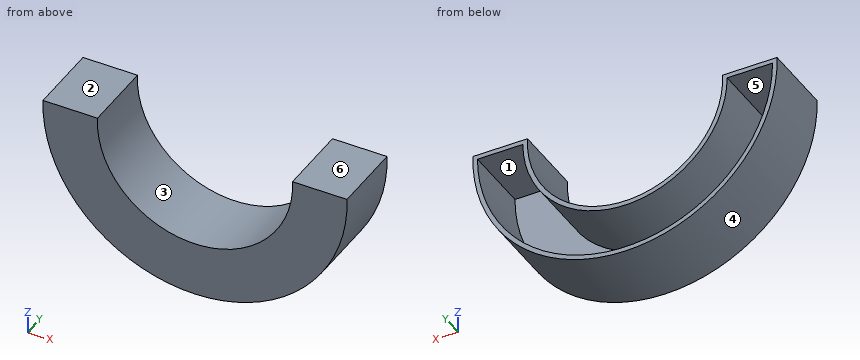
from build123d import *

# Parameters (mm, degrees)
BOSS_EXTRUDE1_DEPTH = 6
BOSS_EXTRUDE2_DEPTH = 0.4


with BuildPart() as part:
    # Sketch3 → Boss-Extrude1 (new body)
    with BuildSketch(Plane(origin=(0, 0, 0), x_dir=(1, 0, 0), z_dir=(0, 1, 0))):
        with BuildLine():
            Line((8.590692638, -0.4), (13.39402852, -0.4))
            ThreePointArc((13.39402852, -0.4), (0, 13.4), (-13.39402852, -0.4))
            Line((-13.39402852, -0.4), (-8.590692638, -0.4))
            ThreePointArc((-8.590692638, -0.4), (0, 8.6), (8.590692638, -0.4))
        make_face()
        with BuildLine():
            Line((9, 0), (13, 0))
            ThreePointArc((13, 0), (0, 13), (-13, 0))
            Line((-13, 0), (-9, 0))
            ThreePointArc((-9, 0), (0, 9), (9, 0))
        make_face(mode=Mode.SUBTRACT)
    extrude(amount=BOSS_EXTRUDE1_DEPTH)

    # Sketch4 → Boss-Extrude2 (add)
    with BuildSketch(Plane.XZ):
        with BuildLine():
            Line((8.590692638, 0.4), (13.39402852, 0.4))
            ThreePointArc((13.39402852, 0.4), (0, -13.4), (-13.39402852, 0.4))
            Line((-13.39402852, 0.4), (-8.590692638, 0.4))
            ThreePointArc((-8.590692638, 0.4), (0, -8.6), (8.590692638, 0.4))
        make_face()
    extrude(amount=BOSS_EXTRUDE2_DEPTH)


solid = part.part
Design review of the part built by this model. Coordinates are the model's own, in mm. Face numbers are marked on the shaded views. A direction names the side the tool comes from. Coordinates: 2 decimals unless noted, no trailing zeros. Write each loop counter-clockwise with the first axis right and the second up, starting at its lowest first coordinate (ties: lowest second). Pieces come first, ordered by that corner, then holes. Notation, with made-up numbers: (54, 83) - (62, 83) arc R16 cw to (62, 89) - close; hole circle Ø9 at (28, 79.25). An arc over 180 degrees is marked (long way). Use one line per item in the form item = value.
Q1. Consider section C-C (x = 0). Write out the cut boundary in (y, z), plus the area to 3 significant figures.
Taken from the geometry:
outline = (-0.4, -13.4) - (6, -13.4) - (6, -13) - (0, -13) - (0, -9) - (6, -9) - (6, -8.6) - (-0.4, -8.6) - close
area = 6.72 mm^2
Q2. Machinability: for the marked faces 5 and 6, which of the approach directions +Z, -Z, +X, -X, +Y, -Y give a long, thin tool a straight path to every point of the face, cutting with its end or side? Answer none if there is none.
Taken from the geometry:
face_5 = +Y
face_6 = +Z, +X, -X, +Y, -Y
Q3. For probe 1 along Z at (x, y) = (0.25, 1); probe 2 along X at (y, z) = (3.25, -7.25); probe 3 along X at (y, z) = (2, -3.25), list the stretches that pass through material, from the lowest coordinate up.
Taken from the geometry:
probe_1 = -13.4 to -13, -9 to -8.6
probe_2 = -11.27 to -10.79, -5.33 to -4.63, 4.63 to 5.33, 10.79 to 11.27
probe_3 = -13 to -12.59, -8.39 to -7.96, 7.96 to 8.39, 12.59 to 13
Q4. Consider section A-A (z = -3.75). Write out the cut boundary in (x, y), plus the area to 3 significant figures.
Taken from the geometry:
outline = (-12.86, -0.4) - (-7.74, -0.4) - (-7.74, 6) - (-8.18, 6) - (-8.18, 0) - (-12.45, 0) - (-12.45, 6) - (-12.86, 6) - close; (7.74, -0.4) - (12.86, -0.4) - (12.86, 6) - (12.45, 6) - (12.45, 0) - (8.18, 0) - (8.18, 6) - (7.74, 6) - close
area = 14.4 mm^2
Q5. The part is to be moulded in two halves that separate along X. For the marked faces 1, 2, 3 and 4, say which applies: +X half, -X half, draft (parallel to the pull), parting line (faces both ways), or undercut.
Taken from the geometry:
face_1 = undercut
face_2 = draft
face_3 = undercut
face_4 = parting line
Q6. Consider section D-D (z = -0.25). Write out the cut boundary in (x, y), plus the area to 3 significant figures.
Taken from the geometry:
outline = (-13.4, -0.4) - (-8.6, -0.4) - (-8.6, 6) - (-9, 6) - (-9, 0) - (-13, 0) - (-13, 6) - (-13.4, 6) - close; (8.6, -0.4) - (13.4, -0.4) - (13.4, 6) - (13, 6) - (13, 0) - (9, 0) - (9, 6) - (8.6, 6) - close
area = 13.4 mm^2
Q7. Insertion check: pin 1 Ø2 at (x, y) = (-11, 3.5) entering from -Z; pin 2 Ø3 at (x, y) = (-2, 4.5) entering from -Z; pin 3 Ø1.5 at (x, z) = (10, -3.5) entering from +Y. Each pin has a flat end and moves straight along its axis. Give the tip position at first contact, or say it passes through.
Taken from the geometry:
pin_1 = -8.92
pin_2 = -13.39
pin_3 = 0
